```python
from build123d import *

# Parameters (mm, degrees)
SKETCH7_R           = 1.5
BOSS_EXTRUDE1_DEPTH = 5
SKETCH8_R           = 17.6
CUT_EXTRUDE1_DEPTH  = 5
FILLET1_R           = 3


with BuildPart() as part:
    # Sketch7 → Boss-Extrude1 (new body)
    with BuildSketch(Plane(origin=(0, -10, 0), x_dir=(1, 0, 0), z_dir=(0, 1, 0))):
        Polygon((80.901699437, 26.286555606), (0, 85.065080835), (-80.901699437, 26.286555606), (-50, -68.819096024), (50, -68.819096024), align=None)
        with Locations((62.122151912, -20.184710728)):
            Circle(SKETCH7_R, mode=Mode.SUBTRACT)
        with Locations((47.457101152, -65.319096024)):
            Circle(SKETCH7_R, mode=Mode.SUBTRACT)
        with Locations((0, -65.319096024)):
            Circle(SKETCH7_R, mode=Mode.SUBTRACT)
        with Locations((-47.457101152, -65.319096024)):
            Circle(SKETCH7_R, mode=Mode.SUBTRACT)
        with Locations((-62.122151912, -20.184710728)):
            Circle(SKETCH7_R, mode=Mode.SUBTRACT)
        with Locations((-76.787202671, 24.949674567)):
            Circle(SKETCH7_R, mode=Mode.SUBTRACT)
        with Locations((-38.393601336, 52.84425874)):
            Circle(SKETCH7_R, mode=Mode.SUBTRACT)
        with Locations((0, 80.738842914)):
            Circle(SKETCH7_R, mode=Mode.SUBTRACT)
        with Locations((76.787202671, 24.949674567)):
            Circle(SKETCH7_R, mode=Mode.SUBTRACT)
        with Locations((38.393601336, 52.84425874)):
            Circle(SKETCH7_R, mode=Mode.SUBTRACT)
    extrude(amount=BOSS_EXTRUDE1_DEPTH)

    # Sketch8 → Cut-Extrude1 (cut)
    with BuildSketch(Plane(origin=(0, -5, 0), x_dir=(1, 0, 0), z_dir=(0, 1, 0))):
        Circle(SKETCH8_R)
    extrude(amount=-CUT_EXTRUDE1_DEPTH, mode=Mode.SUBTRACT)

    # Fillet1
    fillet1_edges = [part.edges().sort_by_distance(p)[0] for p in [
        (50, -7.5, 68.819096024),
        (-50, -7.5, 68.819096024),
        (-80.901699437, -7.5, -26.286555606),
        (0, -7.5, -85.065080835),
        (80.901699437, -7.5, -26.286555606),
    ]]
    fillet(fillet1_edges, radius=FILLET1_R)


solid = part.part
```
Geometry check sheet. Reference: the model listing, model coordinates, mm. Round coordinates to 2 decimals unless told otherwise and drop trailing zeros. Order: outer loops, then holes, each group sorted by start corner. A loop starts at its lowest first (then second) coordinate and runs counter-clockwise, first axis right, second up. Notation, with made-up numbers: M 83,-5 L 139,-5 A31 ccw 139,22 Z; hole C -37,56 d6. An arc over 180 degrees is marked long. Write item = value, one per line.
Q1. Section check A-A (z = 0). Enter the section's corners in (x, y).
Answer block:
outline = M -72.36,-10 L -17.6,-10 L -17.6,-5 L -72.36,-5 Z; M 17.6,-10 L 72.36,-10 L 72.36,-5 L 17.6,-5 Z
Q2. Section check B-B (y = -8.05). Give the number of separate pieces and of enclosed holes in the cut face, plus the area to 3 significant figures.
Answer block:
separate_pieces = 1
enclosed_holes = 11
area = 16,200 mm^2
Q3. Scan lines: line 1 (Z direction, x = 0, y = -8.9); line 2 (X direction, y = -7.3, z = -52.5); line 3 (Z direction, x = -46.5, y = -6.6). Record each from-to range of solid material in increasing order.
Answer block:
line_1 = -84.36 to -82.24, -79.24 to -17.6, 17.6 to 63.82, 66.82 to 68.82
line_2 = -44.82 to -39.85, -36.93 to 36.93, 39.85 to 44.82
line_3 = -51.28 to 64.16, 66.47 to 68.82
Q4. Section check C-C (x = -56.5). Enter the section's corners in (y, z).
Answer block:
outline = M -10,-44.02 L -5,-44.02 L -5,48.81 L -10,48.81 Z
Q5. Depth check by flat-ended pin: pin 1 Ø1 at (y, z) = (-6, -9.5) entering from -X; pin 2 Ø2 at (x, y) = (26.5, -9) entering from -Z. Enter the tip coordinate at first touch or a pass-through.
Answer block:
pin_1 = -75.61
pin_2 = -66.54
Q6. Release check for a two-part mould opening along X. For faces 1 (the flat face through (17, -10, -9)), 2 (the cylindrical face through (16.787, -7.465, -5.287)), 3 (the flat face through (-39.91, -7.54, -56.07)) record: released by +X, released by -X, zero draft, split by the parting line, or undercut.
Answer block:
face_1 = zero draft
face_2 = undercut
face_3 = released by -X
Q7. Section check D-D (z = -44). Enter the section's corners in (x, y).
Answer block:
outline = M -56.52,-10 L 56.52,-10 L 56.52,-5 L -56.52,-5 Z
